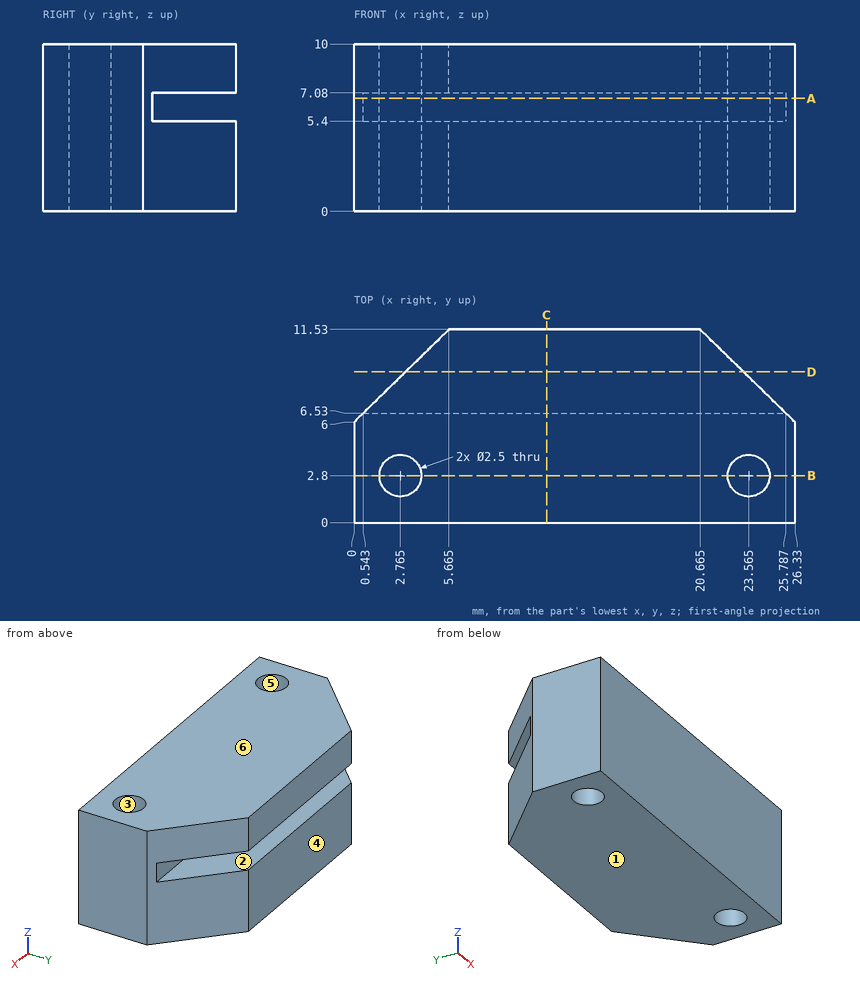
Here's the drawing with two shaded views (mm, measured from the low corner). I have some questions. A direction names the side the tool comes from. Give positions to 0.01 mm unless a question says otherwise; leave off trailing zeros. Order: outer loops, then holes, each group sorted by start corner. A loop starts at its lowest first (then second) coordinate and runs counter-clockwise, first axis right, second up. Notation, with made-up numbers: (45, 64) - (61, 64) arc R6 ccw to (61, 75) - close; hole circle Ø2 at (-30.75, 26.25). An arc over 180 degrees is marked (long way). Write each question's results on one line, items separated by ' | '.
1) Suppose I cut it at B-B, the plane y = 2.8. Write out the boundary of the cut face in (x, z) (3 decimals).
Final values:
outline: (0, 0) - (1.515, 0) - (1.515, 10) - (0, 10) - close; (4.015, 0) - (22.315, 0) - (22.315, 10) - (4.015, 10) - close; (24.815, 0) - (26.33, 0) - (26.33, 10) - (24.815, 10) - close
2) Suppose I cut it at A-A, the plane z = 6.75. Write out the boundary of the cut face in (x, y) (3 decimals), then the cut area to 3 significant figures.
Final values:
outline: (0, 0) - (26.33, 0) - (26.33, 6) - (25.787, 6.53) - (0.543, 6.53) - (0, 6) - close; hole circle Ø2.5 at (2.765, 2.8); hole circle Ø2.5 at (23.565, 2.8) | area: 162 mm^2
3) If we mould it in two halves opening along Y, with no side actions, what happens to the marked faces 3, 4, 5 and 6? For each: pulls with the +Y half, pulls with the -Y half, needs draft (parallel to the pull), parting line crosses it, or undercut.
Final values:
face 3: undercut | face 4: pulls with the +Y half | face 5: undercut | face 6: needs draft
4) Please list where these lines run through material, in increasing order: line 1 along Z through (x, y) = (21, 8); line 2 along X through (y, z) = (2.25, 2.25); line 3 along Y through (x, z) = (2.75, 7). Write a range as [from, to].
Final values:
line 1: z = [0, 5.4], [7.08, 10] | line 2: x = [0, 1.64], [3.89, 22.44], [24.69, 26.33] | line 3: y = [0, 1.55], [4.05, 6.53]
5) On a 3-axis mill with a long thin cutter (end or side, diameter ignored), from which of +Z, -Z, +X, -X, +Y, -Y can I reach the whole of each face in a straight line? I mean the marked faces 1 and 2. Say none if no direction works.
Final values:
face 1: -Z, +X, -X, +Y, -Y | face 2: +X, -X, +Y
6) I'm going to push flat-ended pins straight in: pin 1 Ø2.5 at (x, y) = (19, 9.5) entering from -Z; pin 2 Ø1.5 at (y, z) = (7.5, 5) entering from +X; pin 3 Ø1.5 at (y, z) = (10, 6) entering from -X; pin 4 Ø2 at (x, y) = (23.565, 2.8) entering from -Z. Where does each tip first touch, or does it pass through?
Final values:
pin 1: stops at z = 0 | pin 2: stops at x = 25.56 | pin 3: stops at x = 3.64 | pin 4: passes through
7) Suppose I cut it at D-D, the plane y = 9. Write out the boundary of the cut face in (x, z).
Final values:
outline: (3.07, 0) - (23.26, 0) - (23.26, 5.4) - (3.07, 5.4) - close; (3.07, 7.08) - (23.26, 7.08) - (23.26, 10) - (3.07, 10) - close
8) Suppose I cut it at C-C, the plane x = 11.5. Write out the boundary of the cut face in (y, z).
Final values:
outline: (0, 0) - (11.53, 0) - (11.53, 5.4) - (6.53, 5.4) - (6.53, 7.08) - (11.53, 7.08) - (11.53, 10) - (0, 10) - close
